Design review of the part shown in the three views and the two pictorial views. Dimensions are in mm from the part's minimum x, y and z. A direction names the side the tool comes from. Give positions to 0.01 mm unless a question says otherwise; leave off trailing zeros. Order: outer loops, then holes, each group sorted by start corner. A loop starts at its lowest first (then second) coordinate and runs counter-clockwise, first axis right, second up. Notation, with made-up numbers: (-37.75, -35.5) - (-14.75, -35.5) arc R14 ccw to (-14.75, -17.5) - close; hole circle Ø8 at (26, -39). An arc over 180 degrees is marked (long way). Put each result on its own line as item: value.
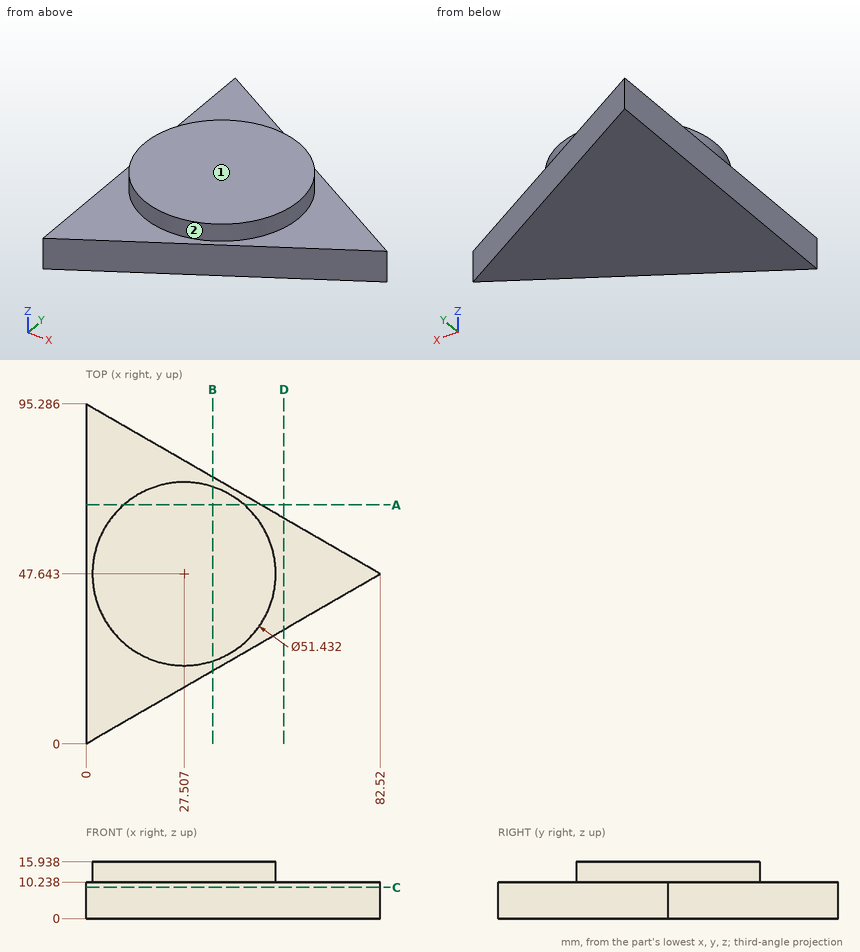
(1) Take a section at D-D, the plane x = 55.5. Write out the cut boundary in (y, z).
The answers:
outline: (32.04, 0) - (63.24, 0) - (63.24, 10.24) - (32.04, 10.24) - close
(2) Clearance check with a flat-ended pin moving along its axis: pin 1 Ø6 at (x, y) = (30, 77.5) entering from +Z. State where the tip first meets the part, or that it passes through.
The answers:
pin 1: z = 10.24
(3) Take a section at C-C, the plane z = 8.75. Write out the cut boundary in (x, y) (1 decimal), then the cut area to 3 significant figures.
The answers:
outline: (0, 0) - (82.5, 47.6) - (0, 95.3) - close
area: 3,930 mm^2
(4) Take a section at A-A, the plane y = 67. Write out the cut boundary in (x, z).
The answers:
outline: (0, 0) - (48.99, 0) - (48.99, 10.24) - (44.44, 10.24) - (44.44, 15.94) - (10.58, 15.94) - (10.58, 10.24) - (0, 10.24) - close
(5) Wall thickness on L1, parallel to X at y = 42.5, z = 14; L2, parallel to Y at x = 51, z = 8.5 (1 decimal); L3, parallel to Y at x = 10.5, z = 6.25 (1 decimal): over which ranges is each line inside the solid? List them lowest first.
The answers:
L1: 2.31 to 52.7
L2: 29.4 to 65.8
L3: 6.1 to 89.2
(6) Take a section at B-B, the plane x = 35.5. Write out the cut boundary in (y, z) (1 decimal).
The answers:
outline: (20.5, 0) - (74.8, 0) - (74.8, 10.2) - (72.1, 10.2) - (72.1, 15.9) - (23.2, 15.9) - (23.2, 10.2) - (20.5, 10.2) - close
(7) For the marked faces 1 and 2, list the 3-axis set-ups (+Z, -Z, +X, -X, +Y, -Y) from which the entire face can be reached by the end or side of a thin tool; tool diameter is ignored.
The answers:
face 1: +Z, +X, -X, +Y, -Y
face 2: +Z
